from build123d import *

# Parameters (mm, degrees)
BOSS_EXTRUDE2_DEPTH = 6.35


with BuildPart() as part:
    # Sketch4 → Boss-Extrude2 (new body)
    with BuildSketch(Plane(origin=(0, 0, 0), x_dir=(1, 0, 0), z_dir=(0, 1, 0))):
        Polygon((-428.205616447, 90.176116322), (-421.855616447, 101.17463895), (-257.614523887, 6.349999946), (-1e-09, 6.35), (1e-09, -6.35), (-261.017478725, -6.35), align=None)
        Polygon((-396.37217922, 75.463246979), (-374.375133964, 62.763246979), (-371.200133964, 68.262508293), (-393.19717922, 80.962508293), align=None, mode=Mode.SUBTRACT)
        Polygon((-313.88325951, 27.838246978), (-291.886214254, 15.138246977), (-288.711214254, 20.637508291), (-310.70825951, 33.337508292), align=None, mode=Mode.SUBTRACT)
        Polygon((-255.913065771, 3.174999946), (-255.913065769, -3.175000054), (-230.513065769, -3.175000048), (-230.513065771, 3.174999952), align=None, mode=Mode.SUBTRACT)
        Polygon((-209.427839463, 3.174999956), (-209.427839461, -3.175000044), (-184.027839461, -3.175000038), (-184.027839463, 3.174999962), align=None, mode=Mode.SUBTRACT)
        Polygon((-120.527839461, -3.175000025), (-120.527839463, 3.174999975), (-145.927839463, 3.174999969), (-145.927839461, -3.175000031), align=None, mode=Mode.SUBTRACT)
        Polygon((-99.442613155, 3.174999979), (-99.442613153, -3.175000021), (-74.042613153, -3.175000015), (-74.042613155, 3.174999985), align=None, mode=Mode.SUBTRACT)
        Polygon((-10.542613153, -3.175000002), (-10.542613155, 3.174999998), (-35.942613155, 3.174999993), (-35.942613153, -3.175000007), align=None, mode=Mode.SUBTRACT)
    extrude(amount=BOSS_EXTRUDE2_DEPTH)


solid = part.part
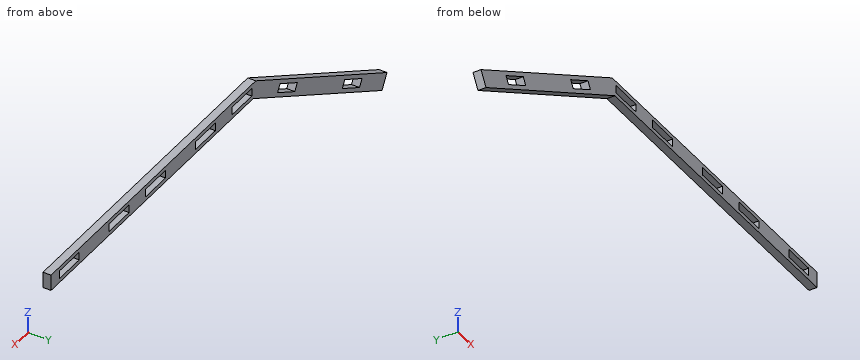
Design review of the part built by this model. Coordinates are the model's own, in mm. Give positions to 0.01 mm unless a question says otherwise; leave off trailing zeros. Loops run counter-clockwise (first coordinate to the right, second up) from the corner with the lowest first, then second, coordinate; pieces in that order, holes last. Notation, with made-up numbers: (75.25, 4.5) - (124.25, 4.5) arc R15 ccw to (124.25, 28.5) - close; hole circle Ø8 at (23.25, 53). An arc over 180 degrees is marked (long way). Write item = value, one per line.
1) Take a section at C-C on x = -61. State the section outline as (y, z) points.
Result sheet:
outline = (0, -6.35) - (6.35, -6.35) - (6.35, 6.35) - (0, 6.35) - close
2) To check wall thickness, follow line 1 (Z direction, x = -136, y = 5) (3 decimals); line 2 (Z direction, x = -50, y = 1.75); line 3 (X direction, y = 4.5, z = -16). State the ranges of each line that lie inside material, in increasing order.
Result sheet:
line_1 = -6.35 to -3.175, 3.175 to 6.35
line_2 = -6.35 to 6.35
line_3 = -299.73 to -293.38, -291.39 to -274.33
3) Take a section at B-B on y = 3.5. Count the separate pieces of the cut face and the enclosed holes in it, and give its area (3 significant figures).
Result sheet:
separate_pieces = 1
enclosed_holes = 7
area = 4,590 mm2
4) Take a section at A-A on x = -252. State the section outline as (y, z) points (3 decimals), and give its area (3 significant figures).
Result sheet:
outline = (0, -6.35) - (6.35, -6.35) - (6.35, -3.175) - (0, -3.175) - close; (0, 3.175) - (6.35, 3.175) - (6.35, 6.35) - (0, 6.35) - close
area = 40.3 mm2
5) Take a section at D-D on z = -54. State the section outline as (x, y) points.
Result sheet:
outline = (-365.55, 0) - (-340.15, 0) - (-340.15, 6.35) - (-365.55, 6.35) - close
6) Clearance check with flat-ended pins moving along their axes: pin 1 Ø1 at (y, z) = (5, -41) entering from -X; pin 2 Ø3 at (y, z) = (5.5, -14) entering from +X; pin 3 Ø3 at (y, z) = (3.5, 0.5) entering from -X. State where each tip first meets the part, or that it passes through.
Result sheet:
pin_1 = -343.9
pin_2 = -268.27
pin_3 = -273.75
